```python
from build123d import *

# Parameters (mm, degrees)
CROQUIS1_W              = 250
CROQUIS1_H              = 250
SALIENTE_EXTRUIR1_DEPTH = 2
CROQUIS2_W              = 8
CROQUIS2_H              = 5
SALIENTE_EXTRUIR2_DEPTH = 6
CROQUIS3_W              = 5
CROQUIS3_H              = 6
SALIENTE_EXTRUIR3_DEPTH = 10
CROQUIS4_W              = 6
CROQUIS4_H              = 5
SALIENTE_EXTRUIR4_DEPTH = 10
CORTAR_EXTRUIR1_REACH   = 187.864
CROQUIS5_R              = 0.983022383
CORTAR_EXTRUIR2_REACH   = 186.678
CROQUIS6_W              = 10
CROQUIS6_H              = 1


with BuildPart() as part:
    # Croquis1 → Saliente-Extruir1 (new body)
    with BuildSketch(Plane(origin=(0, 0, 0), x_dir=(1, 0, 0), z_dir=(0, 1, 0))):
        Rectangle(CROQUIS1_W, CROQUIS1_H)
    extrude(amount=SALIENTE_EXTRUIR1_DEPTH)

    # Croquis2 → Saliente-Extruir2 (add)
    with BuildSketch(Plane(origin=(0, 2, 0), x_dir=(1, 0, 0), z_dir=(0, 1, 0))):
        with Locations((121, 0)):
            Rectangle(CROQUIS2_W, CROQUIS2_H)
    extrude(amount=SALIENTE_EXTRUIR2_DEPTH)

    # Croquis3 → Saliente-Extruir3 (add)
    with BuildSketch(Plane(origin=(125, 0, 0), x_dir=(0, 0, -1), z_dir=(1, 0, 0))):
        with Locations((0, 5)):
            Rectangle(CROQUIS3_W, CROQUIS3_H)
    extrude(amount=SALIENTE_EXTRUIR3_DEPTH)

    # Croquis4 → Saliente-Extruir4 (add)
    with BuildSketch(Plane.XZ.offset(-2)):
        with Locations((132, 0)):
            Rectangle(CROQUIS4_W, CROQUIS4_H)
    extrude(amount=SALIENTE_EXTRUIR4_DEPTH)

    # Croquis5 → Cortar-Extruir1 (cut, up to next)
    with BuildSketch(Plane(origin=(0, 0, -2.5), x_dir=(-1, 0, 0), z_dir=(0, 0, -1)), mode=Mode.PRIVATE) as cortar_extruir1_sk1:
        with Locations((-131, -4)):
            Circle(CROQUIS5_R)
    cortar_extruir1_tool1 = extrude(cortar_extruir1_sk1.sketch, amount=-CORTAR_EXTRUIR1_REACH, mode=Mode.PRIVATE) & part.part
    add(cortar_extruir1_tool1.solids().sort_by_distance((131, -4, -2.5))[0], mode=Mode.SUBTRACT)

    # Croquis6 → Cortar-Extruir2 (cut, up to next)
    with BuildSketch(Plane(origin=(0, 8, 0), x_dir=(1, 0, 0), z_dir=(0, 1, 0)), mode=Mode.PRIVATE) as cortar_extruir2_sk1:
        with Locations((130, -2)):
            Rectangle(CROQUIS6_W, CROQUIS6_H)
    cortar_extruir2_tool1 = extrude(cortar_extruir2_sk1.sketch, amount=-CORTAR_EXTRUIR2_REACH, mode=Mode.PRIVATE) & part.part
    # Croquis6 → Cortar-Extruir2 (cut, up to next)
    with BuildSketch(Plane(origin=(0, 8, 0), x_dir=(1, 0, 0), z_dir=(0, 1, 0)), mode=Mode.PRIVATE) as cortar_extruir2_sk2:
        with Locations((130, 2)):
            Rectangle(CROQUIS6_W, CROQUIS6_H)
    cortar_extruir2_tool2 = extrude(cortar_extruir2_sk2.sketch, amount=-CORTAR_EXTRUIR2_REACH, mode=Mode.PRIVATE) & part.part
    add(cortar_extruir2_tool1.solids().sort_by_distance((130, 8, 2))[0], mode=Mode.SUBTRACT)
    add(cortar_extruir2_tool2.solids().sort_by_distance((130, 8, -2))[0], mode=Mode.SUBTRACT)


solid = part.part
```
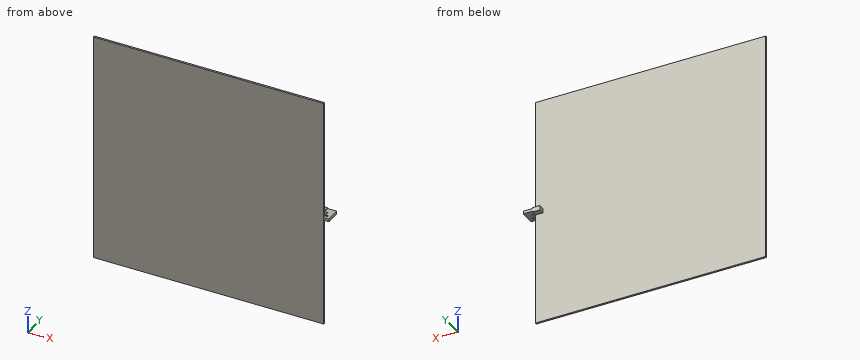
Read the model definition and answer for the solid it produces. Units are mm, in the model's axes. Coordinates: 2 decimals unless noted, no trailing zeros. Write each loop counter-clockwise with the first axis right and the second up, starting at its lowest first coordinate (ties: lowest second). Pieces come first, ordered by that corner, then holes. Notation, with made-up numbers: (-29, 48) - (0, 48) arc R12 cw to (0, 58) - close; hole circle Ø5 at (69, 89.25). An arc over 180 degrees is marked (long way). Answer as a JSON object with one key per item and string values. Group by question number.
1. A cutting plane is placed at B-B (x = -90). Determine the outline of the cut face in (y, z).
2. A cutting plane is placed at A-A (y = 4.75). Determine the outline of the cut face in (x, z), plus the area to 3 significant figures.
3. Each of these flat-tipped pins is pushed along its axis until it touches: P1, Ø5, axis at x = 132, y = -0.5, coming from the +Z side; P2, Ø12, axis at x = -46.5, z = -27.5, coming from the +Y side; P3, Ø6.5, axis at y = 5, z = -37.5, coming from the +X side. Where does it stop, or does it pass through?
4. Consider L1, parallel to Y at x = 131, z = 0; L2, parallel to Y at x = -48.5, z = 97. Determine where each line is inside the solid, lowest interval first. Write a range as [from, to].
5. A cutting plane is placed at C-C (z = -21). Determine the outline of the cut face in (x, y), plus the area to 3 significant figures.
Worked out:
{
 "1": {"outline": "(0, -125) - (2, -125) - (2, 125) - (0, 125) - close"},
 "2": {"outline": "(117, -2.5) - (125, -2.5) - (125, -1.5) - (135, -1.5) - (135, 1.5) - (125, 1.5) - (125, 2.5) - (117, 2.5) - close", "area": "70.0 mm²"},
 "3": {"P1": "stops at z = 1.5", "P2": "stops at y = 2", "P3": "stops at x = 125"},
 "4": {"L1": "y = [-8, -4.98], [-3.02, 8]", "L2": "y = [0, 2]"},
 "5": {"outline": "(-125, 0) - (125, 0) - (125, 2) - (-125, 2) - close", "area": "500 mm²"}
}
